Input: part model. Units: mm. Frame: model coordinates. Face numbers are marked on the shaded views. Coordinates: 2 decimals unless noted, no trailing zeros. Write each loop counter-clockwise with the first axis right and the second up, starting at its lowest first coordinate (ties: lowest second). Pieces come first, ordered by that corner, then holes.
from build123d import *

# Parameters (mm, degrees)
F2_R     = 4
F3_DEPTH = 30
F5_R     = 2.498158
F6_DEPTH = 50


with BuildPart() as f1:
    # F0 (on Front) → F1 (revolve)
    with BuildSketch(Plane.XZ):
        Polygon((-2.5, 0), (0, 0), (0, 1.470086), (-7.284754, 1.470086), align=None)
        Polygon((-5, 0), (-2.5, 0), (-7.284754, 1.470086), (-9.784754, 1.470086), align=None)
        Polygon((-9.784754, 1.470086), (-7.284754, 1.470086), (-37.5, 10.753534), (-40, 10.753534), align=None)
    revolve(axis=Axis((0, 0, 3.122811), (0, 0, 1)))

    # F2 (on face) → F3 (join)
    with BuildSketch(Plane.XY.offset(1.470086)):
        Circle(F2_R)
    extrude(amount=-F3_DEPTH)

    # F5 (on face) → F6 (cut)
    with BuildSketch(Plane(origin=(0, 0, -28.529914), x_dir=(1, 0, 0), z_dir=(0, 0, -1))):
        Circle(F5_R)
    extrude(amount=-F6_DEPTH, mode=Mode.SUBTRACT)


solid = f1.part
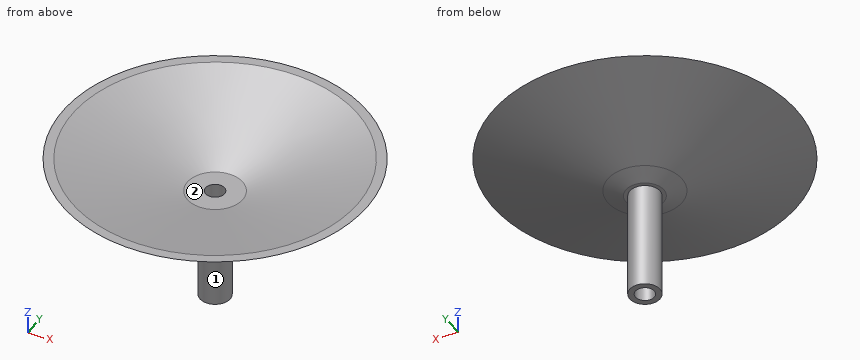
Item 1: Pull-direction query (Y, two-part tool) for the marked faces 1 and 2; classes: released by +Y, released by -Y, zero draft, split by the parting line, or undercut.
Item 2: Section query A-A, the plane z = -9. Return loops of the section in (x, y), then the cut area to 3 significant figures.
Item 3: Material intervals for line 1 (Y direction, x = 0, z = -16); line 2 (Z direction, x = 1, y = -35.5); line 3 (Z direction, x = -27, y = 6), sorted ascending.
Item 4: Pin query (flat end, axial travel): pin 1 Ø4 at (x, y) = (11.5, 24.5) entering from -Z; pin 2 Ø11.5 at (x, y) = (1, 3) entering from +Z; pin 3 Ø1.5 at (x, y) = (-2.5, -1) entering from +Z. Return the tip coordinate at first contact, or that it passes through.
Item 5: Section query B-B, the plane z = 8. Return loops of the section in (x, y).
The answers:
1. face 1: split by the parting line
1. face 2: undercut
2. outline: circle Ø8 at (0, 0); hole circle Ø5 at (0, 0)
2. area: 30.7 mm2
3. line 1: y = -4 to -2.5, 2.5 to 4
3. line 2: z = 9.38 to 10.14
3. line 3: z = 6.96 to 7.73
4. pin 1: stops at z = 6.16
4. pin 2: stops at z = 1.97
4. pin 3: stops at z = 1.47
5. outline: circle Ø62.08 at (0, 0); hole circle Ø57.08 at (0, 0)
